from build123d import *

# Parameters (mm, degrees)
SKETCH1_W           = 800
SKETCH1_H           = 2000
BOSS_EXTRUDE1_DEPTH = 500
SHELL2_T            = -30
SKETCH6_W           = 470
SKETCH6_H           = 5
BOSS_EXTRUDE2_DEPTH = 5
SKETCH8_W           = 470
SKETCH8_H           = 5
BOSS_EXTRUDE3_DEPTH = 5
SKETCH9_W           = 470
SKETCH9_H           = 5
BOSS_EXTRUDE4_DEPTH = 5
SKETCH11_W          = 470
SKETCH11_H          = 5
BOSS_EXTRUDE5_DEPTH = 5
SKETCH16_W          = 470
SKETCH16_H          = 5
BOSS_EXTRUDE6_DEPTH = 5
SKETCH17_W          = 470
SKETCH17_H          = 5
BOSS_EXTRUDE7_DEPTH = 5


with BuildPart() as part:
    # Sketch1 → Boss-Extrude1 (new body)
    with BuildSketch(Plane.XY):
        Rectangle(SKETCH1_W, SKETCH1_H)
    extrude(amount=BOSS_EXTRUDE1_DEPTH)

    # Shell2
    shell2_openings = [part.faces().sort_by_distance(p)[0] for p in [
        (0, 0, 500),
    ]]
    offset(amount=SHELL2_T, openings=shell2_openings, kind=Kind.INTERSECTION)

    # Sketch6 → Boss-Extrude2 (add)
    with BuildSketch(Plane.ZY.offset(-370)):
        with Locations((265, 482.5)):
            Rectangle(SKETCH6_W, SKETCH6_H)
    extrude(amount=BOSS_EXTRUDE2_DEPTH)

    # Sketch8 → Boss-Extrude3 (add)
    with BuildSketch(Plane(origin=(-370, 0, 0), x_dir=(0, 0, -1), z_dir=(1, 0, 0))):
        with Locations((-265, 482.5)):
            Rectangle(SKETCH8_W, SKETCH8_H)
    extrude(amount=BOSS_EXTRUDE3_DEPTH)

    # Sketch9 → Boss-Extrude4 (add)
    with BuildSketch(Plane.ZY.offset(-370)):
        with Locations((265, -2.5)):
            Rectangle(SKETCH9_W, SKETCH9_H)
    extrude(amount=BOSS_EXTRUDE4_DEPTH)

    # Sketch11 → Boss-Extrude5 (add)
    with BuildSketch(Plane(origin=(-370, 0, 0), x_dir=(0, 0, -1), z_dir=(1, 0, 0))):
        with Locations((-265, -2.5)):
            Rectangle(SKETCH11_W, SKETCH11_H)
    extrude(amount=BOSS_EXTRUDE5_DEPTH)

    # Sketch16 → Boss-Extrude6 (add)
    with BuildSketch(Plane.ZY.offset(-370)):
        with Locations((265, -482.5)):
            Rectangle(SKETCH16_W, SKETCH16_H)
    extrude(amount=BOSS_EXTRUDE6_DEPTH)

    # Sketch17 → Boss-Extrude7 (add)
    with BuildSketch(Plane(origin=(-370, 0, 0), x_dir=(0, 0, -1), z_dir=(1, 0, 0))):
        with Locations((-265, -482.5)):
            Rectangle(SKETCH17_W, SKETCH17_H)
    extrude(amount=BOSS_EXTRUDE7_DEPTH)


solid = part.part
Work out the finished part from the listing and answer in its coordinate system (mm). A direction names the side the tool comes from. Give positions to 0.01 mm unless a question says otherwise; leave off trailing zeros. Loops run counter-clockwise (first coordinate to the right, second up) from the corner with the lowest first, then second, coordinate; pieces in that order, holes last. Notation, with made-up numbers: (41.5, 69.25) -> (92.5, 69.25) arc R15 cw to (92.5, 82.25) -> close; hole circle Ø4 at (54.25, 75.5). An arc over 180 degrees is marked (long way). Use a Markdown table: item, result. Add a question column.
1. Flat-ended cylindrical pins translate along their axes: pin 1 Ø5 at (x, y) = (115.5, 265) entering from +Z; pin 2 Ø5 at (x, y) = (-77, 381) entering from -Z. Find the tip coordinate at first contact, or state that the pin passes through.
2. Section B-B on x = -274.5 is taken. Determine the outline of the cut face in (y, z), and give its area (3 significant figures).
3. Find the intervals of material crossed by probe 1 along Y at (x, z) = (-367.5, 454.5); probe 2 along Y at (x, z) = (54, 156.5); probe 3 along X at (y, z) = (441, 143.5), in increasing order.
4. Determine the mould class of faces 1 (the flat face through (-6, 1000, 246)), 2 (the flat face through (-5, -970, 262)), 3 (the flat face through (-6, 14, 0)), 4 (the flat face through (-370, -731, 262)) for opening direction Y: released by +Y, released by -Y, zero draft, split by the parting line, or undercut.
5. For faces 5 (the flat face through (-370, -246, 262)), 6 (the flat face through (400, -14, 246)), determine the directions among +Z, -Z, +X, -X, +Y, -Y from which every point of the face is accessible in a straight line to the end or side of a thin tool.
6. Section C-C on y = 356.5 is taken. Determine the outline of the cut face in (x, z).
Results below:
| question | item | result |
|---|---|---|
| 1 | pin 1 | stops at z = 30 |
| 1 | pin 2 | stops at z = 0 |
| 2 | outline | (-1000, 0) -> (1000, 0) -> (1000, 500) -> (970, 500) -> (970, 30) -> (-970, 30) -> (-970, 500) -> (-1000, 500) -> close |
| 2 | area | 88,200 mm^2 |
| 3 | probe 1 | y = -1000 to -970, -485 to -480, -5 to 0, 480 to 485, 970 to 1000 |
| 3 | probe 2 | y = -1000 to -970, 970 to 1000 |
| 3 | probe 3 | x = -400 to -370, 370 to 400 |
| 4 | face 1 | released by +Y |
| 4 | face 2 | undercut |
| 4 | face 3 | zero draft |
| 4 | face 4 | undercut |
| 5 | face 5 | +Z |
| 5 | face 6 | +Z, -Z, +X, +Y, -Y |
| 6 | outline | (-400, 0) -> (400, 0) -> (400, 500) -> (370, 500) -> (370, 30) -> (-370, 30) -> (-370, 500) -> (-400, 500) -> close |
